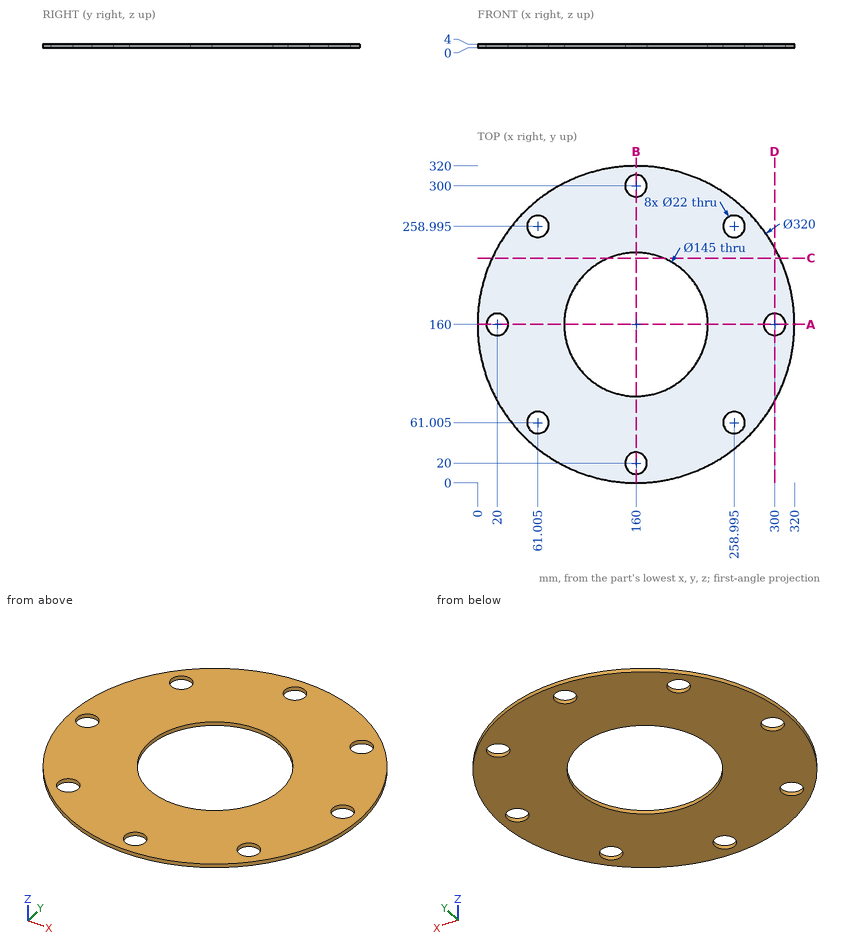
Geometry check sheet. Reference: drawing and pictorial views, mm from the part's lowest x, y, z. Coordinates: 2 decimals unless noted, no trailing zeros. Write each loop counter-clockwise with the first axis right and the second up, starting at its lowest first coordinate (ties: lowest second). Pieces come first, ordered by that corner, then holes. Notation, with made-up numbers: (-26, 57.5) - (17, 57.5) arc R13 ccw to (17, 74.5) - close; hole circle Ø1 at (83, 69). An arc over 180 degrees is marked (long way). One line per question, with ' | ' between items. Start each with the question number.
1. Section check C-C (y = 227). Enter the section's corners in (x, z).
2. Section check D-D (x = 300). Enter the section's corners in (y, z).
3. Section check A-A (y = 160). Enter the section's corners in (x, z), plus the area to 3 significant figures.
4. Gauge pin test, flat ends, axial feed: P1, Ø1, axis at y = 252.5, z = 0.5, coming from the -X side; P2, Ø2, axis at x = 231.5, z = 3, coming from the -Y side. Record the tip position at first contact, or that the pin passes through.
5. Material ranges on line 1 along Y through (x, z) = (160, 2.25); line 2 along Y through (x, z) = (267, 2.7); line 3 along Y through (x, z) = (168.5, 2.2), recorded low to high.
Computed values:
1) outline: (14.7, 0) - (132.3, 0) - (132.3, 4) - (14.7, 4) - close; (187.7, 0) - (305.3, 0) - (305.3, 4) - (187.7, 4) - close
2) outline: (82.54, 0) - (149, 0) - (149, 4) - (82.54, 4) - close; (171, 0) - (237.46, 0) - (237.46, 4) - (171, 4) - close
3) outline: (0, 0) - (9, 0) - (9, 4) - (0, 4) - close; (31, 0) - (87.5, 0) - (87.5, 4) - (31, 4) - close; (232.5, 0) - (289, 0) - (289, 4) - (232.5, 4) - close; (311, 0) - (320, 0) - (320, 4) - (311, 4) - close | area: 524 mm²
4) P1: x = 29.1 | P2: y = 16.37
5) line 1: 0 to 9, 31 to 87.5, 232.5 to 289, 311 to 320 | line 2: 41.04 to 53.46, 68.55 to 251.45, 266.54 to 278.96 | line 3: 0.23 to 13.02, 26.98 to 88, 232 to 293.02, 306.98 to 319.77
